The listing builds one solid part. Answer for the finished solid, in the listing's coordinates (mm). A direction names the side the tool comes from. Coordinates: 2 decimals unless noted, no trailing zeros. Order: outer loops, then holes, each group sorted by start corner. A loop starts at its lowest first (then second) coordinate and runs counter-clockwise, first axis right, second up. Notation, with made-up numbers: (32, -9.75) -> (54, -9.75) arc R19 cw to (54, 9.25) -> close; hole circle Ø4 at (83.5, 53.25). An arc over 180 degrees is marked (long way). Return JSON: item names as keys, results as strings.
```python
from build123d import *

# Parameters (mm, degrees)
SKETCH012_W   = 30
SKETCH012_H   = 50
SKETCH012_R   = 3
SKETCH012_W_2 = 3
SKETCH012_H_2 = 5
PAD012_DEPTH  = 5


with BuildPart() as part:
    # Sketch012 → Pad012 (new body)
    with BuildSketch(Plane(origin=(0, -5, 100), x_dir=(1, 0, 0), z_dir=(0, -1, 0))):
        Rectangle(SKETCH012_W, SKETCH012_H)
        Circle(SKETCH012_R, mode=Mode.SUBTRACT)
        with Locations((-9, 20)):
            Rectangle(SKETCH012_W_2, SKETCH012_H_2, mode=Mode.SUBTRACT)
        with Locations((9, 20)):
            Rectangle(SKETCH012_W_2, SKETCH012_H_2, mode=Mode.SUBTRACT)
        with Locations((-9, -20)):
            Rectangle(SKETCH012_W_2, SKETCH012_H_2, mode=Mode.SUBTRACT)
        with Locations((9, -20)):
            Rectangle(SKETCH012_W_2, SKETCH012_H_2, mode=Mode.SUBTRACT)
    extrude(amount=PAD012_DEPTH)


solid = part.part
```
Item 1: The part is cut by section C-C on z = 81.5. Determine the outline of the cut face in (x, y), plus the area to 3 significant figures.
Answer list:
{"outline": "(-15, -10) -> (-10.5, -10) -> (-10.5, -5) -> (-15, -5) -> close; (-7.5, -10) -> (7.5, -10) -> (7.5, -5) -> (-7.5, -5) -> close; (10.5, -10) -> (15, -10) -> (15, -5) -> (10.5, -5) -> close", "area": "120 mm2"}
Item 2: The part is cut by section D-D on y = -8.9. Determine the outline of the cut face in (x, z), plus the area to 3 significant figures.
Answer list:
{"outline": "(-15, 75) -> (15, 75) -> (15, 125) -> (-15, 125) -> close; hole (-10.5, 77.5) -> (-7.5, 77.5) -> (-7.5, 82.5) -> (-10.5, 82.5) -> close; hole (-10.5, 117.5) -> (-7.5, 117.5) -> (-7.5, 122.5) -> (-10.5, 122.5) -> close; hole circle Ø6 at (0, 100); hole (7.5, 77.5) -> (10.5, 77.5) -> (10.5, 82.5) -> (7.5, 82.5) -> close; hole (7.5, 117.5) -> (10.5, 117.5) -> (10.5, 122.5) -> (7.5, 122.5) -> close", "area": "1,410 mm2"}
Item 3: Which of the six approach directions +Z, -Z, +X, -X, +Y, -Y give full straight-line access (tool end or side, diameter ignored) to faces 1 (the flat face through (15, -7, 100)), 2 (the flat face through (9, -7, 117.5))?
Answer list:
{"face 1": "+Z, -Z, +X, +Y, -Y", "face 2": "+Y, -Y"}
Item 4: The part is cut by section A-A on z = 100. Determine the outline of the cut face in (x, y), plus the area to 3 significant figures.
Answer list:
{"outline": "(-15, -10) -> (-3, -10) -> (-3, -5) -> (-15, -5) -> close; (3, -10) -> (15, -10) -> (15, -5) -> (3, -5) -> close", "area": "120 mm2"}
Item 5: The part is cut by section B-B on x = 0. Determine the outline of the cut face in (y, z).
Answer list:
{"outline": "(-10, 75) -> (-5, 75) -> (-5, 97) -> (-10, 97) -> close; (-10, 103) -> (-5, 103) -> (-5, 125) -> (-10, 125) -> close"}
Item 6: Determine the mould class of faces 3 (the flat face through (0, -7, 125)), 4 (the flat face through (-9, -7, 82.5)), 5 (the flat face through (-15, -7, 100)) for opening direction X: pulls with the +X half, pulls with the -X half, needs draft (parallel to the pull), parting line crosses it, or undercut.
Answer list:
{"face 3": "needs draft", "face 4": "undercut", "face 5": "pulls with the -X half"}
Item 7: Find the intervals of material crossed by probe 1 along Z at (x, y) = (-8, -8.05); probe 2 along X at (y, z) = (-5.7, 78.5); probe 3 along Z at (x, y) = (0, -8.5), in increasing order.
Answer list:
{"probe 1": "75 to 77.5, 82.5 to 117.5, 122.5 to 125", "probe 2": "-15 to -10.5, -7.5 to 7.5, 10.5 to 15", "probe 3": "75 to 97, 103 to 125"}
